Geometry: final body of the model. Coordinates: model frame, mm. Face numbers are marked on the shaded views. A direction names the side the tool comes from. Give positions to 0.01 mm unless a question says otherwise; leave off trailing zeros. Write each loop counter-clockwise with the first axis right and the second up, starting at its lowest first coordinate (ties: lowest second). Pieces come first, ordered by that corner, then holes. Notation, with made-up numbers: (-23.75, 69.5) -> (3.25, 69.5) arc R5 cw to (3.25, 73.5) -> close; hole circle Ø6 at (71.25, 65). An arc over 180 degrees is marked (long way). Use CSV: the item, a comma, the result in double quotes. Start each with the question number.
1) Section B-B (x = 11.5). Output: boundary loops of the cut face in (y, z) (3 decimals), plus the area to 3 significant figures.
2) Section A-A (y = -4). Output: boundary loops of the cut face in (x, z).
3) Section D-D (x = 5). Output: boundary loops of the cut face in (y, z) (3 decimals), plus the area to 3 significant figures.
4) Draft query along Z for the marked faces 4, 5 and 6. Return one class per face: pulls with the +Z half, pulls with the -Z half, needs draft (parallel to the pull), parting line crosses it, or undercut.
5) Contact query for flat-ended pins moving along their axis: P1, Ø1, axis at x = -18, z = 1, coming from the +Y side; P2, Ø1.8, axis at x = 28, z = 4, coming from the +Y side; P3, Ø5, axis at y = -5, z = 9.5, coming from the +X side. Output: stop coordinate, or through.
6) Material intervals for line 1 (Z direction, x = 17.5, y = 2.75); line 2 (Z direction, x = 13.5, y = -3.5); line 3 (Y direction, x = 12.5, z = 1.25) (3 decimals), sorted ascending. Write a range as [from, to].
7) Set-up query: the marked faces 1, 2 and 3. Return all of +Z, -Z, +X, -X, +Y, -Y with unobstructed straight access to the full face (end or side cutting, diameter ignored); none if empty.
8) Section C-C (z = -5). Output: boundary loops of the cut face in (x, y) (3 decimals).
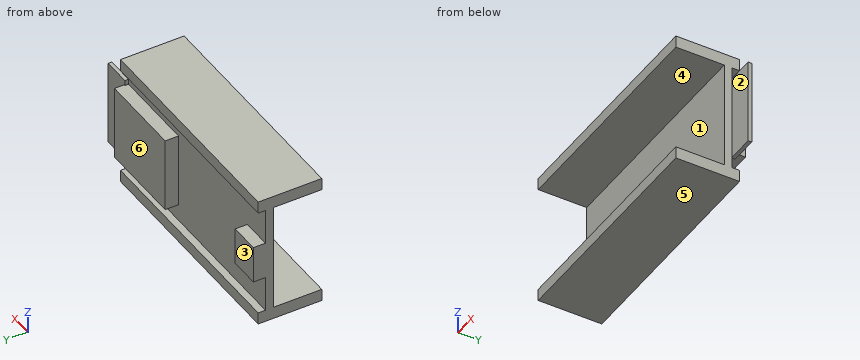
```python
from build123d import *

# Parameters (mm, degrees)
SKETCH1_W                = 48.26
SKETCH1_H                = 27.94
BOSS_EXTRUDE1_DEPTH      = 1.651
BOSS_EXTRUDE2_START      = -11.811
SKETCH2_W                = 48.26
SKETCH2_H                = 2.54
BOSS_EXTRUDE2_DEPTH      = 13.335
SKETCH3_W                = 17.78
SKETCH3_H                = 15.748
BOSS_EXTRUDE3_DEPTH      = 2.794
BOSS_EXTRUDE6_DEPTH      = 5.588
BOSS_EXTRUDE6_DEPTH_BACK = 0.254
SKETCH4_W                = 18.034
SKETCH4_H                = 0.762
SKETCH5_W                = 6.35
SKETCH5_H                = 7.874
BOSS_EXTRUDE7_DEPTH      = 2.54


with BuildPart() as part:
    # Sketch1 → Boss-Extrude1 (new body)
    with BuildSketch(Plane(origin=(0, 0, 0), x_dir=(1, 0, 0), z_dir=(0, 1, 0))):
        Rectangle(SKETCH1_W, SKETCH1_H)
    extrude(amount=BOSS_EXTRUDE1_DEPTH)

    # Sketch2 → Boss-Extrude2 (add)
    with BuildSketch(Plane(origin=(0, 1.651, 0), x_dir=(1, 0, 0), z_dir=(0, 1, 0)).offset(BOSS_EXTRUDE2_START)):
        with Locations((0, -12.7)):
            Rectangle(SKETCH2_W, SKETCH2_H)
    boss_extrude2 = extrude(amount=BOSS_EXTRUDE2_DEPTH)

    # Mirror1: Boss-Extrude2 across plane
    add(boss_extrude2.mirror(Plane.XY))

    # Sketch3 → Boss-Extrude3 (add)
    with BuildSketch(Plane(origin=(0, 1.651, 0), x_dir=(1, 0, 0), z_dir=(0, 1, 0))):
        with Locations((15.24, 0)):
            Rectangle(SKETCH3_W, SKETCH3_H)
    extrude(amount=BOSS_EXTRUDE3_DEPTH)

    # Sketch4 → Boss-Extrude6 (add, two sides: drawn at the far end of the back side and taken through both)
    with BuildSketch(Plane(origin=(24.13, 0, 0), x_dir=(0, 0, -1), z_dir=(1, 0, 0)).offset(-BOSS_EXTRUDE6_DEPTH_BACK)):
        with Locations((0, 2.032)):
            Rectangle(SKETCH4_W, SKETCH4_H)
    extrude(amount=BOSS_EXTRUDE6_DEPTH + BOSS_EXTRUDE6_DEPTH_BACK)

    # Sketch5 → Boss-Extrude7 (add)
    with BuildSketch(Plane(origin=(0, 1.651, 0), x_dir=(1, 0, 0), z_dir=(0, 1, 0))):
        with Locations((-20.955, 0)):
            Rectangle(SKETCH5_W, SKETCH5_H)
    extrude(amount=BOSS_EXTRUDE7_DEPTH)


solid = part.part
```
Answers follow:
1,outline,"(-10.16, -13.97) -> (3.175, -13.97) -> (3.175, -11.43) -> (1.651, -11.43) -> (1.651, -7.874) -> (4.445, -7.874) -> (4.445, 7.874) -> (1.651, 7.874) -> (1.651, 11.43) -> (3.175, 11.43) -> (3.175, 13.97) -> (-10.16, 13.97) -> (-10.16, 11.43) -> (0, 11.43) -> (0, -11.43) -> (-10.16, -11.43) -> close"
1,area,"149 mm^2"
2,outline,"(-24.13, -13.97) -> (24.13, -13.97) -> (24.13, -11.43) -> (-24.13, -11.43) -> close; (-24.13, 11.43) -> (24.13, 11.43) -> (24.13, 13.97) -> (-24.13, 13.97) -> close"
3,outline,"(-10.16, -13.97) -> (3.175, -13.97) -> (3.175, -11.43) -> (1.651, -11.43) -> (1.651, 11.43) -> (3.175, 11.43) -> (3.175, 13.97) -> (-10.16, 13.97) -> (-10.16, 11.43) -> (0, 11.43) -> (0, -11.43) -> (-10.16, -11.43) -> close"
3,area,"105 mm^2"
4,face 4,"undercut"
4,face 5,"pulls with the -Z half"
4,face 6,"needs draft"
5,P1,"stops at y = 4.19"
5,P2,"stops at y = 2.41"
5,P3,"stops at x = 24.13"
6,line 1,"z = [-13.97, -11.43], [-7.87, 7.87], [11.43, 13.97]"
6,line 2,"z = [-13.97, -11.43], [11.43, 13.97]"
6,line 3,"y = [0, 4.445]"
7,face 1,"+X, -X, -Y"
7,face 2,"+Z, -Z, +X, -Y"
7,face 3,"+Z, -Z, -X, +Y"
8,outline,"(-24.13, 0) -> (24.13, 0) -> (24.13, 1.651) -> (29.718, 1.651) -> (29.718, 2.413) -> (24.13, 2.413) -> (24.13, 4.445) -> (6.35, 4.445) -> (6.35, 1.651) -> (-24.13, 1.651) -> close"
